Design review of the part built by this model. Coordinates are the model's own, in mm. Face numbers are marked on the shaded views. A direction names the side the tool comes from. Give positions to 0.01 mm unless a question says otherwise; leave off trailing zeros. Loops run counter-clockwise (first coordinate to the right, second up) from the corner with the lowest first, then second, coordinate; pieces in that order, holes last. Notation, with made-up numbers: (51, 86.5) -> (62, 86.5) arc R25 ccw to (62, 120.5) -> close; hole circle Ø1 at (-12, -17). An arc over 180 degrees is marked (long way). Answer as CSV lines item,"result".
from build123d import *

# Parameters (mm, degrees)
ESQUISSE1_W             = 42
ESQUISSE1_H             = 42
ESQUISSE1_R             = 11.5
ESQUISSE1_R_2           = 1.75
ESQUISSE1_W_2           = 7.5
ESQUISSE1_H_2           = 18
BOSS_EXTRU_1_DEPTH      = 7
ESQUISSE9_R             = 2.25
ENL_V_MAT_EXTRU_2_DEPTH = 17
ENL_V_MAT_EXTRU_3_DEPTH = 4.5
ESQUISSE11_R            = 3.75
ENL_V_MAT_EXTRU_4_DEPTH = 4.5
CONG_1_R                = 5


with BuildPart() as part:
    # Esquisse1 → Boss.-Extru.1 (new body)
    # profile 1 of 2: a face of its own
    with BuildSketch(Plane.XY):
        with Locations((-21, -21)):
            Rectangle(ESQUISSE1_W, ESQUISSE1_H)
        with Locations((-21, -21)):
            Circle(ESQUISSE1_R, mode=Mode.SUBTRACT)
        with Locations((-36.5, -36.5)):
            Circle(ESQUISSE1_R_2, mode=Mode.SUBTRACT)
        with Locations((-5.5, -36.5)):
            Circle(ESQUISSE1_R_2, mode=Mode.SUBTRACT)
        with Locations((-5.5, -5.5)):
            Circle(ESQUISSE1_R_2, mode=Mode.SUBTRACT)
        with Locations((-36.5, -5.611040912)):
            Circle(ESQUISSE1_R_2, mode=Mode.SUBTRACT)
    # profile 2 of 2: a face of its own
    with BuildSketch(Plane.XY):
        with Locations((-45.75, -21)):
            Rectangle(ESQUISSE1_W_2, ESQUISSE1_H_2)
    extrude(amount=BOSS_EXTRU_1_DEPTH)

    # Esquisse9 → Enlèv. mat.-Extru.2 (cut)
    with BuildSketch(Plane.XY.offset(7)):
        with Locations((-44.5, -21)):
            Circle(ESQUISSE9_R)
        with Locations((-37.5, -21)):
            Circle(ESQUISSE9_R)
    extrude(amount=-ENL_V_MAT_EXTRU_2_DEPTH, mode=Mode.SUBTRACT)

    # Esquisse10 → Enlèv. mat.-Extru.3 (cut)
    with BuildSketch(Plane(origin=(0, 0, 0), x_dir=(-1, 0, 0), z_dir=(0, 0, -1))):
        Polygon((44.5, -25.330127019), (48.25, -23.165063509), (48.25, -18.834936491), (44.5, -16.669872981), (40.75, -18.834936491), (40.75, -23.165063509), align=None)
        Polygon((37.5, -25.330127019), (41.25, -23.165063509), (41.25, -18.834936491), (37.5, -16.669872981), (33.75, -18.834936491), (33.75, -23.165063509), align=None)
    extrude(amount=-ENL_V_MAT_EXTRU_3_DEPTH, mode=Mode.SUBTRACT)

    # Esquisse11 → Enlèv. mat.-Extru.4 (cut)
    with BuildSketch(Plane.XY.offset(7)):
        with Locations((-36.5, -5.611040912)):
            Circle(ESQUISSE11_R)
        with Locations((-5.5, -5.5)):
            Circle(ESQUISSE11_R)
        with Locations((-5.5, -36.5)):
            Circle(ESQUISSE11_R)
        with Locations((-36.5, -36.5)):
            Circle(ESQUISSE11_R)
    extrude(amount=-ENL_V_MAT_EXTRU_4_DEPTH, mode=Mode.SUBTRACT)

    # Congé1
    cong_1_edges = [part.edges().sort_by_distance(p)[0] for p in [
        (0, 0, 3.5),
        (0, -42, 3.5),
        (-42, -42, 3.5),
        (-42, 0, 3.5),
    ]]
    fillet(cong_1_edges, radius=CONG_1_R)


solid = part.part
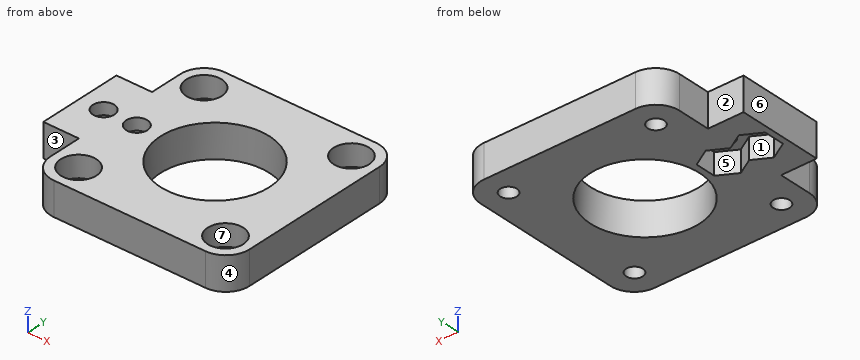
Q1. We need section B-B, the plane x = -46. State the section outline as (y, z) points, and give its area (3 significant figures).
Filled sheet:
outline,"(-30, 0) -> (-24.46, 0) -> (-24.46, 4.5) -> (-22.68, 4.5) -> (-22.68, 7) -> (-30, 7) -> close; (-19.32, 4.5) -> (-17.54, 4.5) -> (-17.54, 0) -> (-12, 0) -> (-12, 7) -> (-19.32, 7) -> close"
area,"86.4 mm^2"
Q2. We need section D-D, the plane z = 1.5. State the section outline as (x, y) points, and give its area (3 significant figures).
Filled sheet:
outline,"(-49.5, -30) -> (-42, -30) -> (-42, -37) arc R5 ccw to (-37, -42) -> (-5, -42) arc R5 ccw to (0, -37) -> (0, -5) arc R5 ccw to (-5, 0) -> (-37, 0) arc R5 ccw to (-42, -5) -> (-42, -12) -> (-49.5, -12) -> close; hole (-48.25, -23.17) -> (-44.5, -25.33) -> (-41, -23.31) -> (-37.5, -25.33) -> (-33.75, -23.17) -> (-33.75, -18.83) -> (-37.5, -16.67) -> (-41, -18.69) -> (-44.5, -16.67) -> (-48.25, -18.83) -> close; hole circle Ø3.5 at (-36.5, -36.5); hole circle Ø3.5 at (-36.5, -5.61); hole circle Ø23 at (-21, -21); hole circle Ø3.5 at (-5.5, -36.5); hole circle Ø3.5 at (-5.5, -5.5)"
area,"1,330 mm^2"
Q3. We need section A-A, the plane y = -21. State the section outline as (x, z) points.
Filled sheet:
outline,"(-49.5, 0) -> (-48.25, 0) -> (-48.25, 4.5) -> (-46.75, 4.5) -> (-46.75, 7) -> (-49.5, 7) -> close; (-42.25, 4.5) -> (-39.75, 4.5) -> (-39.75, 7) -> (-42.25, 7) -> close; (-35.25, 4.5) -> (-33.75, 4.5) -> (-33.75, 0) -> (-32.5, 0) -> (-32.5, 7) -> (-35.25, 7) -> close; (-9.5, 0) -> (0, 0) -> (0, 7) -> (-9.5, 7) -> close"
Q4. The part is to be moulded in two halves that separate along Y. For the marked faces 4, 5, 6 and 7, say which applies: pulls with the +Y half, pulls with the -Y half, needs draft (parallel to the pull), parting line crosses it, or undercut.
Filled sheet:
face 4,"pulls with the -Y half"
face 5,"undercut"
face 6,"needs draft"
face 7,"undercut"
Q5. We need section C-C, the plane y = -26. State the section outline as (x, z) points.
Filled sheet:
outline,"(-49.5, 0) -> (-31.36, 0) -> (-31.36, 7) -> (-49.5, 7) -> close; (-10.64, 0) -> (0, 0) -> (0, 7) -> (-10.64, 7) -> close"
Q6. Clearance check with flat-ended pins moving along their axes: pin 1 Ø4 at (x, y) = (-5, -32.5) entering from -Z; pin 2 Ø1.5 at (x, y) = (-22.5, -10.5) entering from +Z; pin 3 Ø4 at (x, z) = (-40, 3) entering from +Y; pin 4 Ø3.5 at (x, z) = (-47, 2.5) entering from +Y. State where each tip first meets the part, or that it passes through.
Filled sheet:
pin 1,"stops at z = 0"
pin 2,"passes through"
pin 3,"stops at y = -0.1"
pin 4,"stops at y = -12"
Q7. To check wall thickness, follow probe 1 along Y at (x, z) = (-5.5, 4.1); probe 2 along Y at (x, z) = (-5.5, 1.85). State the ranges of each line that lie inside material, in increasing order. Write a range as from..to.
Filled sheet:
probe 1,"y = -42..-40.25, -32.75..-9.25, -1.75..0"
probe 2,"y = -42..-38.25, -34.75..-7.25, -3.75..0"
Q8. For the marked faces 1, 2 and 3, list the 3-axis set-ups (+Z, -Z, +X, -X, +Y, -Y) from which the entire face can be reached by the end or side of a thin tool; tool diameter is ignored.
Filled sheet:
face 1,"-Z"
face 2,"+Z, -Z, -X, +Y"
face 3,"+Z, -Z, -X, -Y"
